Build history of the part. All positions in model axes, mm. Face numbers are marked on the shaded views. A direction names the side the tool comes from. Round coordinates to 2 decimals unless told otherwise and drop trailing zeros. Write each loop counter-clockwise with the first axis right and the second up, starting at its lowest first coordinate (ties: lowest second). Pieces come first, ordered by that corner, then holes. Notation, with made-up numbers: (27.25, -38.75) - (67.25, -38.75) arc R34 cw to (67.25, -8.75) - close; hole circle Ø3 at (-3.5, 54). An arc over 180 degrees is marked (long way). Write each question's results on one line, items separated by ' | '.
from build123d import *

# Parameters (mm, degrees)
EXTRUDE_1_DEPTH    = 200
HOLE_WIZARD_M3_1_D = 2.5


with BuildPart() as part:
    # 草图1 → 拉伸-薄壁1 (new body)
    with BuildSketch(Plane(origin=(0, 0, 0), x_dir=(1, 0, 0), z_dir=(0, 1, 0))):
        with BuildLine():
            Line((400, -24), (0, -24))
            ThreePointArc((0, -24), (-24, 0), (0, 24))
            Line((0, 24), (400, 24))
            ThreePointArc((400, 24), (424, 0), (400, -24))
        make_face()
        with BuildLine():
            Line((400, -20), (0, -20))
            ThreePointArc((0, -20), (-20, 0), (0, 20))
            Line((0, 20), (400, 20))
            ThreePointArc((400, 20), (420, 0), (400, -20))
        make_face(mode=Mode.SUBTRACT)
    extrude(amount=EXTRUDE_1_DEPTH)

    # M3 螺纹孔1 (through all)
    with Locations(Plane.XY.offset(24)):
        with Locations((40.682677542, 140), (40.682677542, 60)):
            Hole(HOLE_WIZARD_M3_1_D / 2)


solid = part.part
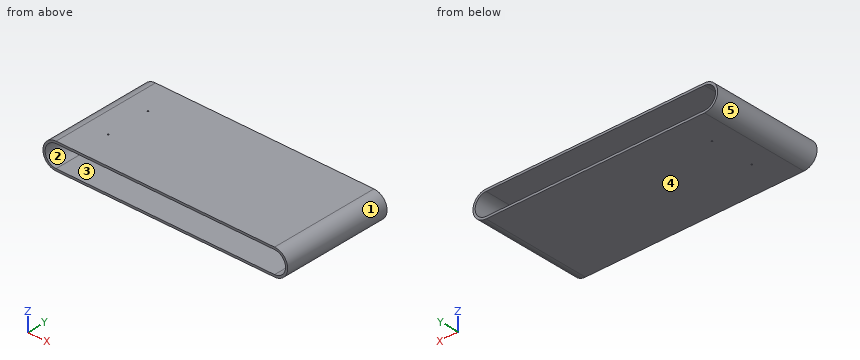
(1) Drill centre lines: probe 1 along Z at (x, y) = (33.5, 184); probe 2 along X at (y, z) = (158, 1); probe 3 along X at (y, z) = (128.5, -9). Where is each one in solid material? Low to high. Write a range as [from, to].
Worked answers:
probe 1: z = [-24, -20], [20, 24] | probe 2: x = [-23.98, -19.97], [419.97, 423.98] | probe 3: x = [-22.25, -17.86], [417.86, 422.25]
(2) Slice it at A-A, the plane x = 381.5. Write the cut outline in (y, z), and give its area (3 significant figures).
Worked answers:
outline: (0, -24) - (200, -24) - (200, -20) - (0, -20) - close; (0, 20) - (200, 20) - (200, 24) - (0, 24) - close | area: 1,600 mm2
(3) Flat gauge pins, fed straight in: pin 1 Ø2 at (x, y) = (40.68, 140) entering from -Z (3 decimals); pin 2 Ø1 at (y, z) = (41, 7) entering from -X; pin 3 Ø3 at (y, z) = (71.5, 8.5) entering from +X; pin 4 Ø1 at (y, z) = (111.5, 14.5) entering from +X. Where does each tip first touch, or does it go through?
Worked answers:
pin 1: passes through | pin 2: stops at x = -23.1 | pin 3: stops at x = 422.96 | pin 4: stops at x = 419.49
(4) Slice it at C-C, the plane y = 76. Write the cut outline in (x, z).
Worked answers:
outline: (0, -24) - (400, -24) arc R24 ccw to (400, 24) - (0, 24) arc R24 ccw to start; hole (0, -20) - (400, -20) arc R20 ccw to (400, 20) - (0, 20) arc R20 ccw to start
(5) Two-plate mould, pull along Z, no slides. Class the marked faces 3, 4 and 5: released by +Z, released by -Z, zero draft, split by the parting line, or undercut.
Worked answers:
face 3: undercut | face 4: released by -Z | face 5: split by the parting line
(6) Tool access for the marked faces 1 and 2: list every direction of +Z, -Z, +X, -X, +Y, -Y with a clear straight run to the whole face (end or side of a thin tool).
Worked answers:
face 1: +X, +Y, -Y | face 2: +Y, -Y
(7) Slice it at B-B, the plane z = 0. Write the cut outline in (x, y), and give its area (3 significant figures).
Worked answers:
outline: (-24, 0) - (-20, 0) - (-20, 200) - (-24, 200) - close; (420, 0) - (424, 0) - (424, 200) - (420, 200) - close | area: 1,600 mm2
